Could you check a few things on this model? Use its own coordinates, in mm. Face numbers are marked on the shaded views. A direction names the side the tool comes from. Give positions to 0.01 mm unless a question says otherwise; leave off trailing zeros. Order: outer loops, then holes, each group sorted by start corner. A loop starts at its lowest first (then second) coordinate and runs counter-clockwise, first axis right, second up. Notation, with made-up numbers: (74.5, 54) - (105.5, 54) arc R22 ccw to (105.5, 85) - close; hole circle Ø3 at (-25, 3.25). An arc over 180 degrees is marked (long way). Put each result on its own line as item: value.
from build123d import *

# Parameters (mm, degrees)
SKETCH1_R                = 6
BOSS_EXTRUDE1_DEPTH      = 4
BOSS_EXTRUDE2_DEPTH      = 4
BOSS_EXTRUDE2_DEPTH_BACK = 8
SKETCH2_R                = 4
SKETCH8_R                = 1.4
SKETCH6_R                = 1.46


with BuildPart() as part:
    # Sketch1 → Boss-Extrude1 (new body)
    with BuildSketch(Plane.XY.offset(33)):
        Circle(SKETCH1_R)
    extrude(amount=-BOSS_EXTRUDE1_DEPTH)

    # Sketch2 → Boss-Extrude2 (add, two sides: drawn at the far end of the back side and taken through both)
    with BuildSketch(Plane.XY.offset(33).offset(-BOSS_EXTRUDE2_DEPTH_BACK)):
        Circle(SKETCH2_R)
    extrude(amount=BOSS_EXTRUDE2_DEPTH + BOSS_EXTRUDE2_DEPTH_BACK)

    # Sketch8 → Cut-Loft2 section 0
    with BuildSketch(Plane.XY.offset(37)):
        Circle(SKETCH8_R)
    # Sketch6 → Cut-Loft2 section 1
    with BuildSketch(Plane.XY.offset(25)):
        Circle(SKETCH6_R)
    loft(mode=Mode.SUBTRACT)


solid = part.part
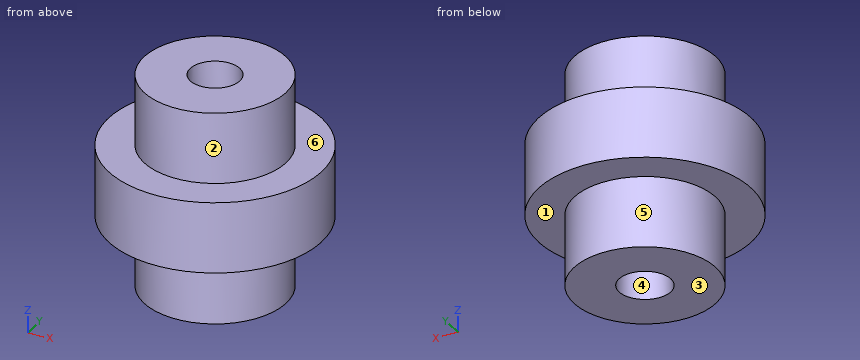
1) Which directions (+Z, -Z, +X, -X, +Y, -Y) give clear straight access to the entire face, cutting with the end or side of a thin tool? Please do the marked faces 1, 2 and 3.
Filled in:
face 1: -Z
face 2: +Z
face 3: -Z, +X, -X, +Y, -Y
2) Suppose I cut it at C-C, the plane z = 36.25. List the corners of the cut face in (x, y) for me.
Filled in:
outline: circle Ø8 at (0, 0); hole circle Ø2.81 at (0, 0)
3) We'd pull the mould along Y, two halves only. Please class the marked faces 4, 5 and 6: pulls with the +Y half, pulls with the -Y half, needs draft (parallel to the pull), parting line crosses it, or undercut.
Filled in:
face 4: undercut
face 5: parting line crosses it
face 6: needs draft
4) I'm going to push flat-ended pins straight in: pin 1 (5 mm diameter, centred on y = -4, z = 30, fed in from +X); pin 2 (1.5 mm diameter, centred on y = -1.5, z = 31, fed in from +X). Where does each tip first touch, or does it pass through?
Filled in:
pin 1: stops at x = 5.81
pin 2: stops at x = 5.95
5) Suppose I cut it at A-A, the plane x = 2. List the corners of the cut face in (y, z) for me.
Filled in:
outline: (-5.66, 29) - (-3.46, 29) - (-3.46, 25) - (3.46, 25) - (3.46, 29) - (5.66, 29) - (5.66, 33) - (3.46, 33) - (3.46, 37) - (-3.46, 37) - (-3.46, 33) - (-5.66, 33) - close
6) Suppose I cut it at D-D, the plane z = 34. List the corners of the cut face in (x, y) for me (3 decimals).
Filled in:
outline: circle Ø8 at (0, 0); hole circle Ø2.83 at (0, 0)
7) Suppose I cut it at B-B, the plane y = -3.5. List the corners of the cut face in (x, z) for me, and give its area (3 significant figures).
Filled in:
outline: (-4.87, 29) - (-1.94, 29) - (-1.94, 25) - (1.94, 25) - (1.94, 29) - (4.87, 29) - (4.87, 33) - (1.94, 33) - (1.94, 37) - (-1.94, 37) - (-1.94, 33) - (-4.87, 33) - close
area: 70.0 mm^2
8) If I drill on line 1 (X direction, y = -0.25, z = 36.75); line 2 (Y direction, x = -1, z = 26.25); line 3 (Y direction, x = -0.25, z = 30.75), over which ranges is the centre line in solid material (lowest first)? Write a range as [from, to].
Filled in:
line 1: x = [-3.99, -1.38], [1.38, 3.99]
line 2: y = [-3.87, -1.06], [1.06, 3.87]
line 3: y = [-5.99, -1.41], [1.41, 5.99]
